For this review, take the finished solid that the model builds, in its own axes (mm). Face numbers are marked on the shaded views. A direction names the side the tool comes from. Coordinates: 2 decimals unless noted, no trailing zeros. Loops run counter-clockwise (first coordinate to the right, second up) from the corner with the lowest first, then second, coordinate; pieces in that order, holes last. Notation, with made-up numbers: M 11.5,36.5 L 22.5,36.5 A28 ccw 22.5,69.5 Z; hole C 31.5,52 d3. An arc over 180 degrees is marked long. Use one line per item in the form item = value.
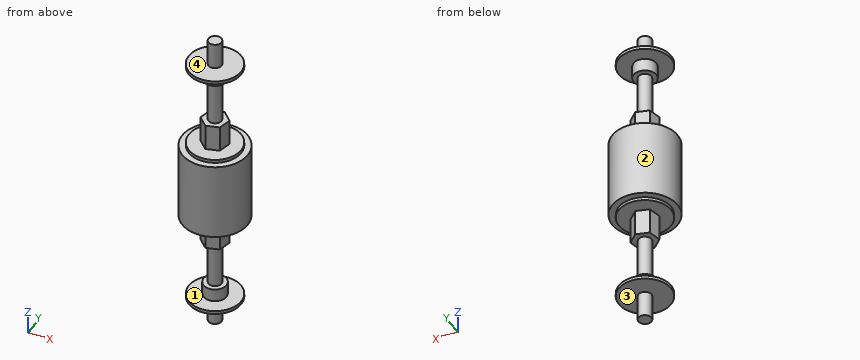
```python
from build123d import *

# Parameters (mm, degrees)
SKETCH1_R           = 15.875
BOSS_EXTRUDE1_DEPTH = 19.05
SKETCH2_R           = 12.7
BOSS_EXTRUDE2_DEPTH = 1.5875
BOSS_EXTRUDE3_DEPTH = 12.7
SKETCH4_R           = 3.175
BOSS_EXTRUDE4_DEPTH = 22.225
SKETCH5_R           = 5.55625
BOSS_EXTRUDE6_DEPTH = 6.35
SKETCH6_R           = 12.7
BOSS_EXTRUDE7_DEPTH = 1.5875
SKETCH7_R           = 3.175
BOSS_EXTRUDE8_DEPTH = 12.7


with BuildPart() as part:
    # Sketch1 → Boss-Extrude1 (new body)
    with BuildSketch(Plane.XY):
        Circle(SKETCH1_R)
    boss_extrude1 = extrude(amount=BOSS_EXTRUDE1_DEPTH)

    # Sketch2 → Boss-Extrude2 (add)
    with BuildSketch(Plane.XY.offset(19.05)):
        Circle(SKETCH2_R)
    boss_extrude2 = extrude(amount=BOSS_EXTRUDE2_DEPTH)

    # Sketch3 → Boss-Extrude3 (add)
    with BuildSketch(Plane.XY.offset(20.6375)):
        Polygon((4.603141218, -4.469188183), (6.17200111, 1.75184314), (1.568859892, 6.221031323), (-4.603141218, 4.469188183), (-6.17200111, -1.75184314), (-1.568859892, -6.221031323), align=None)
    boss_extrude3 = extrude(amount=BOSS_EXTRUDE3_DEPTH)

    # Sketch4 → Boss-Extrude4 (add)
    with BuildSketch(Plane.XY.offset(33.3375)):
        Circle(SKETCH4_R)
    boss_extrude4 = extrude(amount=BOSS_EXTRUDE4_DEPTH)

    # Sketch5 → Boss-Extrude6 (add)
    with BuildSketch(Plane.XY.offset(55.5625)):
        Circle(SKETCH5_R)
    boss_extrude6 = extrude(amount=BOSS_EXTRUDE6_DEPTH)

    # Sketch6 → Boss-Extrude7 (add)
    with BuildSketch(Plane.XY.offset(61.9125)):
        Circle(SKETCH6_R)
    boss_extrude7 = extrude(amount=BOSS_EXTRUDE7_DEPTH)

    # Sketch7 → Boss-Extrude8 (add)
    with BuildSketch(Plane.XY.offset(63.5)):
        Circle(SKETCH7_R)
    boss_extrude8 = extrude(amount=BOSS_EXTRUDE8_DEPTH)

    # Mirror1: Boss-Extrude1, Boss-Extrude2, Boss-Extrude3, Boss-Extrude4, Boss-Extrude6, Boss-Extrude7, Boss-Extrude8 across plane
    add(boss_extrude1.mirror(Plane.XY))
    add(boss_extrude2.mirror(Plane.XY))
    add(boss_extrude3.mirror(Plane.XY))
    add(boss_extrude4.mirror(Plane.XY))
    add(boss_extrude6.mirror(Plane.XY))
    add(boss_extrude7.mirror(Plane.XY))
    add(boss_extrude8.mirror(Plane.XY))


solid = part.part
```
1. Consider section A-A on y = -8. Write out the cut boundary in (x, z).
Computed values:
outline = M -13.71,-19.05 L -9.86,-19.05 L -9.86,-20.64 L 9.86,-20.64 L 9.86,-19.05 L 13.71,-19.05 L 13.71,19.05 L 9.86,19.05 L 9.86,20.64 L -9.86,20.64 L -9.86,19.05 L -13.71,19.05 Z; M -9.86,-63.5 L 9.86,-63.5 L 9.86,-61.91 L -9.86,-61.91 Z; M -9.86,61.91 L 9.86,61.91 L 9.86,63.5 L -9.86,63.5 Z
2. Tool access review of the marked faces 1, 2, 3 and 4: name each direction out of +Z, -Z, +X, -X, +Y, -Y from which nothing blocks a thin tool from reaching the whole face with its end or side.
Computed values:
face_1 = none
face_2 = +Z, -Z
face_3 = -Z
face_4 = +Z
3. Consider section C-C on z = -25.5. Write out the cut boundary in (x, y), plus the area to 3 significant figures.
Computed values:
outline = M -6.17,-1.75 L -1.57,-6.22 L 4.6,-4.47 L 6.17,1.75 L 1.57,6.22 L -4.6,4.47 Z
area = 107 mm2
4. For pin 1 Ø5 at (x, z) = (2, -50.5) entering from -Y (3 decimals); pin 2 Ø12 at (y, z) = (11.5, 3) entering from +X; pin 3 Ø1.5 at (x, z) = (-8.5, 12) entering from -Y; pin 4 Ø16 at (x, y) = (-7, -6.5) entering from +Z, all flat-tipped, find the tip position at first contact; note any pin that passes through.
Computed values:
pin_1 = -3.175
pin_2 = 14.89
pin_3 = -13.85
pin_4 = 76.2
5. Consider section D-D on z = -41. Write out the cut boundary in (x, y) (3 decimals), plus the area to 3 significant figures.
Computed values:
outline = C 0,0 d6.35
area = 31.7 mm2
6. Wall thickness on line 1 along Z through (x, y) = (-7, -10); line 2 along Z through (x, y) = (-2, 3.5); line 3 along Z through (x, y) = (11, 7): over which ranges is each line inside the solid? List them lowest first. Write a range as from..to.
Computed values:
line_1 = -63.5..-61.91, -20.64..20.64, 61.91..63.5
line_2 = -63.5..-55.56, -33.34..33.34, 55.56..63.5
line_3 = -19.05..19.05
7. Consider section B-B on x = 9.5. Write out the cut boundary in (y, z), plus the area to 3 significant figures.
Computed values:
outline = M -12.72,-19.05 L -8.43,-19.05 L -8.43,-20.64 L 8.43,-20.64 L 8.43,-19.05 L 12.72,-19.05 L 12.72,19.05 L 8.43,19.05 L 8.43,20.64 L -8.43,20.64 L -8.43,19.05 L -12.72,19.05 Z; M -8.43,-63.5 L 8.43,-63.5 L 8.43,-61.91 L -8.43,-61.91 Z; M -8.43,61.91 L 8.43,61.91 L 8.43,63.5 L -8.43,63.5 Z
area = 1,080 mm2
